```python
from build123d import *

# Parameters (mm, degrees)
SKETCH1_W           = 100
SKETCH1_H           = 20
BOSS_EXTRUDE1_DEPTH = 6
FILLET1_R           = 10
SKETCH2_R           = 5
CUT_EXTRUDE1_DEPTH  = 103.156742313


with BuildPart() as part:
    # Sketch1 → Boss-Extrude1 (new body)
    with BuildSketch(Plane(origin=(0, 0, 0), x_dir=(1, 0, 0), z_dir=(0, 1, 0))):
        with Locations((50, 10)):
            Rectangle(SKETCH1_W, SKETCH1_H)
    extrude(amount=BOSS_EXTRUDE1_DEPTH)

    # Fillet1
    fillet1_edges = [part.edges().sort_by_distance(p)[0] for p in [
        (100, 3, -20),
        (100, 3, 0),
        (0, 3, -20),
        (0, 3, 0),
    ]]
    fillet(fillet1_edges, radius=FILLET1_R - 0.0001)  # a hair under: the kernel refuses the full size

    # Sketch2 → Cut-Extrude1 (cut, through all)
    with BuildSketch(Plane(origin=(0, 6, 0), x_dir=(1, 0, 0), z_dir=(0, 1, 0))):
        with Locations(Location((10, 10, 0), (0, 0, 270))):
            Circle(SKETCH2_R)
        with Locations(Location((90, 10, 0), (0, 0, 270))):
            Circle(SKETCH2_R)
    extrude(amount=-CUT_EXTRUDE1_DEPTH, mode=Mode.SUBTRACT)


solid = part.part
```
Could you check a few things on this model? Use its own coordinates, in mm. Coordinates: 2 decimals unless noted, no trailing zeros. Write each loop counter-clockwise with the first axis right and the second up, starting at its lowest first coordinate (ties: lowest second). Pieces come first, ordered by that corner, then holes. Notation, with made-up numbers: (30.25, 21.25) -> (79.25, 21.25) arc R34 cw to (79.25, 51.25) -> close; hole circle Ø5 at (74.25, -18). An arc over 180 degrees is marked (long way). One line per question, with ' | ' between items. Start each with the question number.
1. Will these pins go through, and if not, where does the flat tip stop? P1, Ø1, axis at y = 2, z = -15, coming from the -X side; P2, Ø1.5, axis at y = 1.5, z = -5, coming from the -X side.
2. Thinking about a two-plate mould opening in Z: for faces 1 (the face through (11.5, 3.04, -5.23)), 2 (the face through (2.85, 3.04, -3.01)), 3 (the face through (49, 6, -10)), which applies, pulls with the +Z half, pulls with the -Z half, needs draft (parallel to the pull), parting line crosses it, or undercut?
3. If we section it at D-D (z = -18): Please give me the cut outline in (x, y).
4. If we section it at B-B (z = -7): Please give me the cut outline in (x, y), and give its area (3 significant figures).
5. If we section it at A-A (y = 1.1): Count the separate pieces of the cut face and the enclosed holes in it, and give its area (3 significant figures).
6. If we section it at C-C (z = -13.5): Please give me the cut outline in (x, y).
7. Please list where these lines run through material, in increasing order: line 1 along X through (y, z) = (3.7, -10); line 2 along X through (y, z) = (4.1, -8); line 3 along Z through (x, y) = (89, 0.9).
Return value:
1) P1: stops at x = 1.07 | P2: stops at x = 0.95
2) face 1: undercut | face 2: pulls with the +Z half | face 3: needs draft
3) outline: (4, 0) -> (96, 0) -> (96, 6) -> (4, 6) -> close
4) outline: (0.46, 0) -> (6, 0) -> (6, 6) -> (0.46, 6) -> close; (14, 0) -> (86, 0) -> (86, 6) -> (14, 6) -> close; (94, 0) -> (99.54, 0) -> (99.54, 6) -> (94, 6) -> close | area: 498 mm²
5) separate pieces: 1 | enclosed holes: 2 | area: 1,760 mm²
6) outline: (0.63, 0) -> (6.43, 0) -> (6.43, 6) -> (0.63, 6) -> close; (13.57, 0) -> (86.43, 0) -> (86.43, 6) -> (13.57, 6) -> close; (93.57, 0) -> (99.37, 0) -> (99.37, 6) -> (93.57, 6) -> close
7) line 1: x = 0 to 5, 15 to 85, 95 to 100 | line 2: x = 0.2 to 5.42, 14.58 to 85.42, 94.58 to 99.8 | line 3: z = -20 to -14.9, -5.1 to 0
